Check sheet for the modelled part. Datum: model origin and axes. Units: mm. Give positions to 0.01 mm unless a question says otherwise; leave off trailing zeros. Loops run counter-clockwise (first coordinate to the right, second up) from the corner with the lowest first, then second, coordinate; pieces in that order, holes last. Notation, with made-up numbers: M 19,87.5 L 64,87.5 A20 ccw 64,100.5 Z; hole C -10,38.25 d8. An arc over 180 degrees is marked long. Use one line per item in the form item = value.
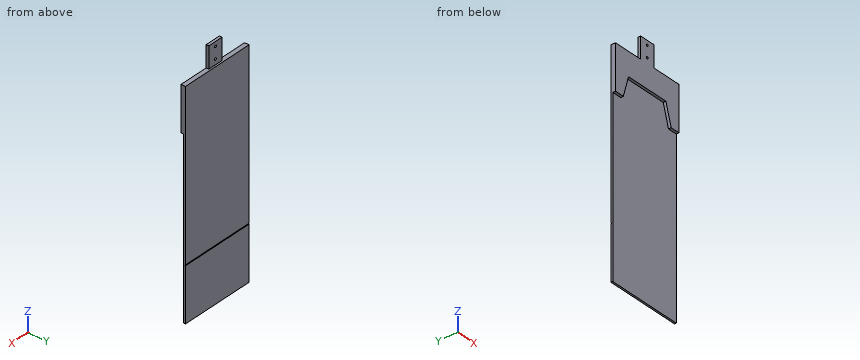
from build123d import *

# Parameters (mm, degrees)
BOSS_EXTRUDE1_DEPTH                  = 3
SKETCH10_W                           = 17.5
SKETCH10_H                           = 24
BOSS_EXTRUDE2_DEPTH                  = 3
F_2_5_2_5_DIAMETER_HOLE1_D           = 2.5
F_2_5_2_5_DIAMETER_HOLE1_DEPTH       = 6.35
F_2_5_2_5_DIAMETER_HOLE1_CSINK_D     = 2.55
F_2_5_2_5_DIAMETER_HOLE1_CSINK_ANGLE = 90
F_2_5_2_5_DIAMETER_HOLE1_TIP         = 0.751075774
CUT_EXTRUDE3_DEPTH                   = 4
SKETCH11_W                           = 85
SKETCH11_H                           = 245
BOSS_EXTRUDE3_DEPTH                  = 2
SKETCH12_W                           = 1
SKETCH12_H                           = 0.5
CUT_EXTRUDE4_DEPTH                   = 1
CUT_EXTRUDE4_DEPTH_BACK              = 86


with BuildPart() as part:
    # Sketch2 → Boss-Extrude1 (new body)
    with BuildSketch(Plane(origin=(0, 0, 0), x_dir=(1, 0, 0), z_dir=(0, 1, 0))):
        Polygon((42.5, 0), (42.5, 50), (22.5, 50), (8.75, 26.184301396), (-8.75, 26.184301396), (-22.5, 50), (-42.5, 50), (-42.5, 0), align=None)
    extrude(amount=BOSS_EXTRUDE1_DEPTH)

    # Sketch10 → Boss-Extrude2 (add)
    with BuildSketch(Plane(origin=(0, 3, 0), x_dir=(1, 0, 0), z_dir=(0, 1, 0))):
        with Locations((0, -12)):
            Rectangle(SKETCH10_W, SKETCH10_H)
    extrude(amount=-BOSS_EXTRUDE2_DEPTH)

    # Ø2.5 (2.5) Diameter Hole1
    with Locations(Plane(origin=(0, 3, 0), x_dir=(1, 0, 0), z_dir=(0, 1, 0))):
        with Locations((0, -19), (0, -6)):
            CounterSinkHole(F_2_5_2_5_DIAMETER_HOLE1_D / 2, F_2_5_2_5_DIAMETER_HOLE1_CSINK_D / 2, depth=F_2_5_2_5_DIAMETER_HOLE1_DEPTH, counter_sink_angle=F_2_5_2_5_DIAMETER_HOLE1_CSINK_ANGLE)
            with Locations((0, 0, -(F_2_5_2_5_DIAMETER_HOLE1_DEPTH + F_2_5_2_5_DIAMETER_HOLE1_TIP / 2))):  # 118° drill point
                Cone(0, F_2_5_2_5_DIAMETER_HOLE1_D / 2, F_2_5_2_5_DIAMETER_HOLE1_TIP, mode=Mode.SUBTRACT)

    # Sketch9 → Cut-Extrude3 (cut, through all)
    with BuildSketch(Plane.XZ):
        Polygon((-32, -50), (-25, -26.184301396), (25, -26.184301396), (32, -50), align=None)
    extrude(amount=-CUT_EXTRUDE3_DEPTH, mode=Mode.SUBTRACT)

    # Sketch11 → Boss-Extrude3 (add)
    with BuildSketch(Plane(origin=(0, 3, 0), x_dir=(1, 0, 0), z_dir=(0, 1, 0))):
        with Locations((0, 122.5)):
            Rectangle(SKETCH11_W, SKETCH11_H)
    extrude(amount=BOSS_EXTRUDE3_DEPTH)

    # Sketch12 → Cut-Extrude4 (cut, two sides)
    with BuildSketch(Plane.ZY.offset(42.5)) as cut_extrude4_sk:
        with Locations((-184.5, 4.75)):
            Rectangle(SKETCH12_W, SKETCH12_H)
    extrude(amount=CUT_EXTRUDE4_DEPTH, mode=Mode.SUBTRACT)
    extrude(cut_extrude4_sk.sketch, amount=-CUT_EXTRUDE4_DEPTH_BACK, mode=Mode.SUBTRACT)


solid = part.part
1) Section check D-D (x = -27.5). Record the cut outline in (y, z), then the cut area to 3 significant figures.
Evaluation:
outline = M 0,-34.69 L 3,-34.69 L 3,-245 L 5,-245 L 5,-185 L 4.5,-185 L 4.5,-184 L 5,-184 L 5,0 L 0,0 Z
area = 594 mm^2
2) Depth check by flat-ended pin: pin 1 Ø3 at (x, z) = (0, 19) entering from +Y; pin 2 Ø1.5 at (x, y) = (-6.5, 1.5) entering from -Z; pin 3 Ø2.5 at (y, z) = (1, 10.5) entering from +X. Enter the tip coordinate at first touch or a pass-through.
Evaluation:
pin_1 = 3
pin_2 = -26.18
pin_3 = 8.75
3) Section check C-C (z = -46.5). Record the cut outline in (x, y).
Evaluation:
outline = M -42.5,0 L -30.97,0 L -30.97,3 L 30.97,3 L 30.97,0 L 42.5,0 L 42.5,5 L -42.5,5 Z
4) Section check B-B (y = 1.8). Record the cut outline in (x, z).
Evaluation:
outline = M -42.5,-50 L -32,-50 L -25,-26.18 L 25,-26.18 L 32,-50 L 42.5,-50 L 42.5,0 L 8.75,0 L 8.75,24 L -8.75,24 L -8.75,0 L -42.5,0 Z; hole C 0,6 d2.5; hole C 0,19 d2.5
5) Section check A-A (x = -4.5). Record the cut outline in (y, z).
Evaluation:
outline = M 0,-26.18 L 3,-26.18 L 3,-245 L 5,-245 L 5,-185 L 4.5,-185 L 4.5,-184 L 5,-184 L 5,0 L 3,0 L 3,24 L 0,24 Z
6) Scan lines: line 1 (Z direction, x = 0, y = 1.9); line 2 (X direction, y = 1.95, z = 6); line 3 (Y direction, x = -7.5, z = -69). Record each from-to range of solid material in increasing order.
Evaluation:
line_1 = -26.18 to 4.75, 7.25 to 17.75, 20.25 to 24
line_2 = -8.75 to -1.25, 1.25 to 8.75
line_3 = 3 to 5
